Study the drawing (mm; zero at the part's minimum x, y, z) and answer. A direction names the side the tool comes from. Round coordinates to 2 decimals unless told otherwise and drop trailing zeros. Write each loop counter-clockwise with the first axis right and the second up, starting at its lowest first coordinate (ties: lowest second). Pieces come first, ordered by that corner, then holes.
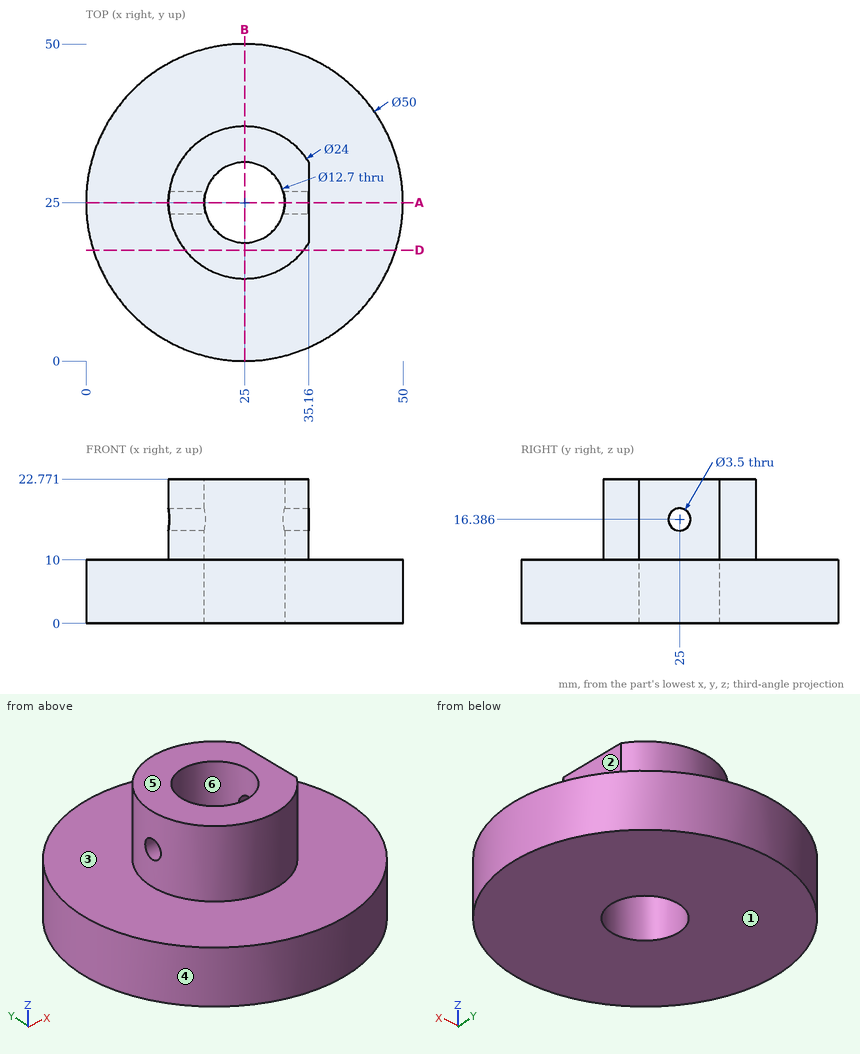
Q1. Find section B-B (x = 25). Determine the outline of the cut face in (y, z), plus the area to 3 significant figures.
Q2. The mould has two halves that part along Y. Classify the marked faces 4, 5 and 6: +Y half, -Y half, draft (parallel to the pull), parting line (faces both ways), or undercut.
Q3. Given pin 1 (4 mm diameter, centred on x = 8, z = 6, fed in from +Y); pin 2 (8 mm diameter, centred on y = 23, z = 17.5, fed in from +X); pin 3 (5 mm diameter, centred on x = 26, y = 7.5, fed in from +Z); pin 4 (11.5 mm diameter, centred on x = 25, y = 25, fed in from +Z), each flat-ended and moving along its own axis, determine where each tip first touches the part or whether it passes through.
Q4. A tool of negligible diameter and unlimited length cuts with its end or side. For the marked faces 1, 2 and 3, from which of +Z, -Z, +X, -X, +Y, -Y can it reach the whole face along a straight path? Write none if from no direction.
Q5. Find the intervals of material crossed by L1, parallel to X at y = 25, z = 11; L2, parallel to Y at x = 25, z = 12.5; L3, parallel to Z at x = 33.1, y = 25 (1 decimal), in increasing order.
Q6. Find section A-A (y = 25). Count the separate pieces of the cut face and the enclosed holes in it, plus the area to 3 significant figures.
Q7. Find section D-D (y = 17.5). Determine the outline of the cut face in (x, z), plus the area to 3 significant figures.
Report:
1. outline: (0, 0) - (18.65, 0) - (18.65, 22.77) - (13, 22.77) - (13, 10) - (0, 10) - close; (31.35, 0) - (50, 0) - (50, 10) - (37, 10) - (37, 22.77) - (31.35, 22.77) - close
1. area: 517 mm2
2. face 4: parting line
2. face 5: draft
2. face 6: undercut
3. pin 1: stops at y = 45
3. pin 2: stops at x = 35.16
3. pin 3: stops at z = 10
3. pin 4: passes through
4. face 1: -Z, +X, -X, +Y, -Y
4. face 2: +Z, +X, +Y, -Y
4. face 3: +Z
5. L1: x = 13 to 18.65, 31.35 to 35.16
5. L2: y = 13 to 18.65, 31.35 to 37
5. L3: z = 0 to 14.6, 18.1 to 22.8
6. separate pieces: 4
6. enclosed holes: 0
6. area: 461 mm2
7. outline: (1.15, 0) - (48.85, 0) - (48.85, 10) - (34.37, 10) - (34.37, 22.77) - (15.63, 22.77) - (15.63, 10) - (1.15, 10) - close
7. area: 716 mm2
